from build123d import *

# Parameters (mm, degrees)
F1_DEPTH = 75
F2_R     = 0.3
F3_R     = 10
F4_R     = 5
F6_R     = 3.25
F7_DEPTH = 25
F8_R     = 5
F8_R_2   = 3.25
F9_DEPTH = 6


with BuildPart() as f1:
    # F0 (on Front) → F1 (new body)
    with BuildSketch(Plane.XZ):
        Polygon((-20.15, 4.595843), (-12, 5.5), (12, 5.5), (20.15, 4.595843), (20.15, 0), (17.384257, -2.674988), (24.15, -2.674988), (24.15, 0), (24.15, 15), (-24.15, 15), (-24.15, 0), (-24.15, -2.674988), (-17.384257, -2.674988), (-20.15, 0), align=None)
    extrude(amount=F1_DEPTH)

    # F2
    f2_edges = [f1.edges().sort_by_distance(p)[0] for p in [
        (-17.384257, -37.5, -2.674988),
        (17.384257, -37.5, -2.674988),
    ]]
    fillet(f2_edges, radius=F2_R)

    # F3
    f3_edges = [f1.edges().sort_by_distance(p)[0] for p in [
        (-24.15, -37.5, 15),
        (24.15, -37.5, 15),
    ]]
    fillet(f3_edges, radius=F3_R)

    # F4
    f4_edges = [f1.edges().sort_by_distance(p)[0] for p in [
        (-24.15, -37.5, -2.674988),
        (24.15, -37.5, -2.674988),
    ]]
    fillet(f4_edges, radius=F4_R)


with BuildPart() as f1_1:
    # F5: moved
    add(f1.part.moved(Location((0, 37.5, 0))))

    # F6 (on face) → F7 (cut)
    with BuildSketch(Plane.XY.offset(15)):
        with Locations((0, 27)):
            Circle(F6_R)
        with Locations((0, -27)):
            Circle(F6_R)
    extrude(amount=-F7_DEPTH, mode=Mode.SUBTRACT)

    # F8 (on face) → F9 (cut)
    with BuildSketch(Plane.XY.offset(15)):
        with Locations((0, 27)):
            Circle(F8_R)
        with Locations((0, 27)):
            Circle(F8_R_2, mode=Mode.SUBTRACT)
        with Locations((0, -27)):
            Circle(F8_R)
        with Locations((0, -27)):
            Circle(F8_R_2, mode=Mode.SUBTRACT)
    extrude(amount=-F9_DEPTH, mode=Mode.SUBTRACT)


with BuildPart() as f1_2:
    # F10: moved
    add(f1_1.part.moved(Location((0, 0, -15))))


solid = f1_2.part
Could you check a few things on this model? Use its own coordinates, in mm. A direction names the side the tool comes from. Coordinates: 2 decimals unless noted, no trailing zeros. Write each loop counter-clockwise with the first axis right and the second up, starting at its lowest first coordinate (ties: lowest second). Pieces come first, ordered by that corner, then holes. Notation, with made-up numbers: (-33.75, -24) - (-22.75, -24) arc R29 cw to (-22.75, 7) - close; hole circle Ø2 at (34.5, 12.5). An arc over 180 degrees is marked (long way). Put each result on its own line as item: value. Start each with the question number.
Q1. I want a section at D-D on z = -15.75. Write out the boundary of the cut face in (x, y), plus the area to 3 significant figures.
Q2. I want a section at A-A on y = 27. Write out the boundary of the cut face in (x, z), plus the area to 3 significant figures.
Q3. I'm going to push flat-ended pins straight in: P1, Ø5, axis at x = 0, y = 27, coming from the -Z side; P2, Ø1.5, axis at y = 9.5, z = -9, coming from the +X side; P3, Ø2, axis at y = -3.5, z = -3, coming from the +X side; P4, Ø19, axis at x = 0, y = -3, coming from the -Z side. Where does each tip first touch, or does it pass through?
Q4. I want a section at C-C on y = 10.5. Write out the boundary of the cut face in (x, z), plus the area to 3 significant figures.
Q5. I want a section at B-B on x = 0. Write out the boundary of the cut face in (y, z), plus the area to 3 significant figures.
Q6. Please list where these lines run through material, in increasing order: L1, parallel to Y at x = 0, z = -7.75; L2, parallel to Y at x = 0, z = -3.05; L3, parallel to Z at x = -9.5, y = -31.5.
Q7. Thinking about a two-plate mould opening in Y: for faces 4 (the flat face through (0, 37.5, -7)), 5 (the cylindrical face through (-0.705, 23.827, -7.726)), 6 (the flat face through (0, 1, -9.5)), 7 (the cylindrical face through (-1.08, 22.12, -2.96)), which applies, pulls with the +Y half, pulls with the -Y half, needs draft (parallel to the pull), parting line crosses it, or undercut?
Q8. Which directions (+Z, -Z, +X, -X, +Y, -Y) give clear straight access to the entire face, cutting with the end or side of a thin tool? Please do faces 1 (the flat face through (-19.018, 0.525, -16.095)), 2 (the cylindrical face through (-1.08, -31.88, -2.96)), 3 (the flat face through (24.15, 1, -11)).
Checks:
1. outline: (-23.09, -37.5) - (-19.37, -37.5) - (-19.37, 37.5) - (-23.09, 37.5) - close; (19.37, -37.5) - (23.09, -37.5) - (23.09, 37.5) - (19.37, 37.5) - close
1. area: 558 mm²
2. outline: (-24.15, -12.67) arc R5 ccw to (-19.15, -17.67) - (-18.13, -17.67) arc R0.3 ccw to (-17.92, -17.16) - (-20.15, -15) - (-20.15, -10.4) - (-12, -9.5) - (-3.25, -9.5) - (-3.25, -6) - (-5, -6) - (-5, 0) - (-14.15, 0) arc R10 ccw to (-24.15, -10) - close; (3.25, -9.5) - (12, -9.5) - (20.15, -10.4) - (20.15, -15) - (17.92, -17.16) arc R0.3 ccw to (18.13, -17.67) - (19.15, -17.67) arc R5 ccw to (24.15, -12.67) - (24.15, -10) arc R10 ccw to (14.15, 0) - (5, 0) - (5, -6) - (3.25, -6) - close
2. area: 402 mm²
3. P1: through
3. P2: x = 24.15
3. P3: x = 22.15
3. P4: z = -9.5
4. outline: (-24.15, -12.67) arc R5 ccw to (-19.15, -17.67) - (-18.13, -17.67) arc R0.3 ccw to (-17.92, -17.16) - (-20.15, -15) - (-20.15, -10.4) - (-12, -9.5) - (12, -9.5) - (20.15, -10.4) - (20.15, -15) - (17.92, -17.16) arc R0.3 ccw to (18.13, -17.67) - (19.15, -17.67) arc R5 ccw to (24.15, -12.67) - (24.15, -10) arc R10 ccw to (14.15, 0) - (-14.15, 0) arc R10 ccw to (-24.15, -10) - close
4. area: 485 mm²
5. outline: (-37.5, -9.5) - (-30.25, -9.5) - (-30.25, -6) - (-32, -6) - (-32, 0) - (-37.5, 0) - close; (-23.75, -9.5) - (23.75, -9.5) - (23.75, -6) - (22, -6) - (22, 0) - (-22, 0) - (-22, -6) - (-23.75, -6) - close; (30.25, -9.5) - (37.5, -9.5) - (37.5, 0) - (32, 0) - (32, -6) - (30.25, -6) - close
5. area: 547 mm²
6. L1: -37.5 to -30.25, -23.75 to 23.75, 30.25 to 37.5
6. L2: -37.5 to -32, -22 to 22, 32 to 37.5
6. L3: -9.5 to 0
7. face 4: pulls with the +Y half
7. face 5: undercut
7. face 6: needs draft
7. face 7: undercut
8. face 1: +Y, -Y
8. face 2: +Z
8. face 3: +Z, -Z, +X, +Y, -Y
